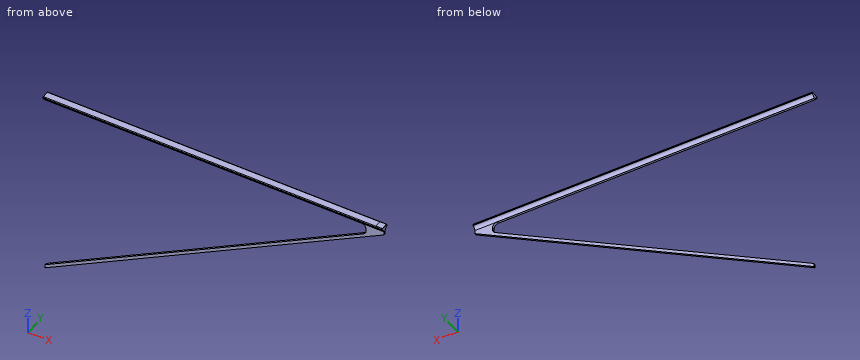
from build123d import *

# Parameters (mm, degrees)
F1_DEPTH      = 502
F3_DEPTH      = 406
F4_DEPTH      = 143
F5_W          = 26.22529459
F5_H          = 3
F6_DEPTH      = 14.25
F6_DEPTH_BACK = 0.8
F8_DEPTH      = 25
F10_DEPTH     = 0.27
F11_R         = 7
F12_R         = 7
F13_T1_DEPTH  = 502
F14_T1_DEPTH  = 502
F15_T1_DEPTH  = 507
F15_T6_DEPTH  = 507
F15_T12_DEPTH = 507
F15_T18_DEPTH = 507
F15_T25_DEPTH = 507
F15_T31_DEPTH = 507


# Not quite as in the source:
# - a fillet or chamfer that OpenCascade refuses, or shapes differently, is made with other operations: its cross-section is extruded or revolved along the edge and cut away or added
# - a feature names something its author has since deleted; it is built from what else it names


with BuildPart() as f1:
    # F0 (on Right) → F1 (new body)
    with BuildSketch(Plane.YZ):
        Polygon((6, 24.6420782059), (-6, 24.6420782059), (-6, 22.1420782059), (-1.5, 22.1420782059), (-1.5, -257.8579217941), (1.5, -257.8579217941), (1.5, 22.1420782059), (6, 22.1420782059), align=None)
    extrude(amount=F1_DEPTH)

    # F2 (on face) → F3 (cut)
    with BuildSketch(Plane.XZ.offset(1.5)):
        Polygon((0, -252.8579217941), (502, 17.1420782059), (0, 17.1420782059), align=None)
    extrude(amount=-F3_DEPTH, mode=Mode.SUBTRACT)

    # F2 (on face) → F4 (cut)
    with BuildSketch(Plane.XZ.offset(1.5)):
        Polygon((502, -257.8579217941), (502, 12.1420782059), (0, -257.8579217941), align=None)
    extrude(amount=-F4_DEPTH, mode=Mode.SUBTRACT)

    # F5 (on face) → F6 (join, two sides)
    with BuildSketch(Plane(origin=(0, 0, 17.1420782059), x_dir=(1, 0, 0), z_dir=(0, 0, -1))) as f6_sk:
        with Locations((488.887352705, 0)):
            Rectangle(F5_W, F5_H)
    extrude(amount=F6_DEPTH)
    extrude(f6_sk.sketch, amount=-F6_DEPTH_BACK)

    # F7 (on face) → F8 (cut)
    with BuildSketch(Plane(origin=(0, 1.5, 0), x_dir=(-1, 0, 0), z_dir=(0, 1, 0))):
        Polygon((-484.8018518519, 2.8920782059), (-502, 12.143202126), (-502, 2.8920782059), align=None)
    extrude(amount=-F8_DEPTH, mode=Mode.SUBTRACT)

    # F9 (on face) → F10 (join)
    with BuildSketch(Plane.XY.offset(24.6420782059)):
        Polygon((501.9800190187, -5.0222751118), (501.9800190187, 4.9777248882), (497.843503952, 4.9777248882), (491.9800190187, 4.9777248882), (491.9800190187, -5.0222751118), (496.5066611767, -5.0222751118), align=None)
    extrude(amount=F10_DEPTH)

    # F11
    f11_edges = [f1.edges().sort_by_distance(p)[0] for p in [
        (475.774705, 0, 17.142078),
    ]]
    fillet(f11_edges, radius=F11_R)

    # F12
    f12_edges = [f1.edges().sort_by_distance(p)[0] for p in [
        (475.774705, 0, 3.03684),
    ]]
    fillet(f12_edges, radius=F12_R)

    # F13: fillet of radius 5 on 1 edges, made by hand

    # F13_s2 → F13_t1 (join)
    with BuildSketch(Plane.YZ):
        with BuildLine():
            ThreePointArc((1.5, 17.1671410204), (2.7919007565, 20.5212429867), (6, 22.1420782059))
            Line((6, 22.1420782059), (1.5, 22.1420782059))
            Line((1.5, 22.1420782059), (1.5, 17.1671410204))
        make_face()
    extrude(amount=F13_T1_DEPTH)

    # F14: fillet of radius 5 on 1 edges, made by hand

    # F14_s2 → F14_t1 (join)
    with BuildSketch(Plane.YZ):
        with BuildLine():
            ThreePointArc((-1.5, 17.1671410204), (-2.7919007565, 20.5212429867), (-6, 22.1420782059))
            Line((-6, 22.1420782059), (-1.5, 22.1420782059))
            Line((-1.5, 22.1420782059), (-1.5, 17.1671410204))
        make_face()
    extrude(amount=F14_T1_DEPTH)

    # F15: fillet of radius 1 on 2 edges, made by hand

    # F15_s2 → F15_t1 (cut)
    with BuildSketch(Plane.YZ.offset(-2.5)):
        with BuildLine():
            ThreePointArc((6, 23.6420782059), (5.7071067812, 24.3491849871), (5, 24.6420782059))
            Line((5, 24.6420782059), (6, 24.6420782059))
            Line((6, 24.6420782059), (6, 23.6420782059))
        make_face()
    extrude(amount=F15_T1_DEPTH, mode=Mode.SUBTRACT)


with BuildPart() as f15_tool4:
    # F15_s5 → F15_t6 (new body)
    with BuildSketch(Plane.YZ.offset(-2.5)):
        with BuildLine():
            ThreePointArc((-5, 24.6420782059), (-5.7071067812, 24.3491849871), (-6, 23.6420782059))
            Line((-6, 23.6420782059), (-6, 24.6420782059))
            Line((-6, 24.6420782059), (-5, 24.6420782059))
        make_face()
    extrude(amount=F15_T6_DEPTH)

    split(bisect_by=Plane.YZ.offset(491.9800190187), keep=Keep.BOTTOM)

    split(bisect_by=Plane.XZ.offset(5.0222751118), keep=Keep.BOTTOM)


with BuildPart() as f1_1:
    add(f1.part)

    # F15_t3: cut F15_tool4
    add(f15_tool4.part, mode=Mode.SUBTRACT)


with BuildPart() as f15_tool10:
    # F15_s11 → F15_t12 (new body)
    with BuildSketch(Plane.YZ.offset(-2.5)):
        with BuildLine():
            ThreePointArc((-5, 24.6420782059), (-5.7071067812, 24.3491849871), (-6, 23.6420782059))
            Line((-6, 23.6420782059), (-6, 24.6420782059))
            Line((-6, 24.6420782059), (-5, 24.6420782059))
        make_face()
    extrude(amount=F15_T12_DEPTH)

    split(bisect_by=Plane.YZ.offset(491.9800190187), keep=Keep.BOTTOM)

    split(bisect_by=Plane.XZ.offset(5.0222751118), keep=Keep.TOP)


with BuildPart() as f1_2:
    add(f1_1.part)

    # F15_t9: cut F15_tool10
    add(f15_tool10.part, mode=Mode.SUBTRACT)


with BuildPart() as f15_tool16:
    # F15_s17 → F15_t18 (new body)
    with BuildSketch(Plane.YZ.offset(-2.5)):
        with BuildLine():
            ThreePointArc((-5, 24.6420782059), (-5.7071067812, 24.3491849871), (-6, 23.6420782059))
            Line((-6, 23.6420782059), (-6, 24.6420782059))
            Line((-6, 24.6420782059), (-5, 24.6420782059))
        make_face()
    extrude(amount=F15_T18_DEPTH)

    split(bisect_by=Plane.YZ.offset(491.9800190187), keep=Keep.TOP)

    split(bisect_by=Plane.YZ.offset(501.9800190187), keep=Keep.BOTTOM)

    split(bisect_by=Plane.XZ.offset(5.0222751118), keep=Keep.TOP)


with BuildPart() as f1_3:
    add(f1_2.part)

    # F15_t15: cut F15_tool16
    add(f15_tool16.part, mode=Mode.SUBTRACT)


with BuildPart() as f15_tool23:
    # F15_s24 → F15_t25 (new body)
    with BuildSketch(Plane.YZ.offset(-2.5)):
        with BuildLine():
            ThreePointArc((-5, 24.6420782059), (-5.7071067812, 24.3491849871), (-6, 23.6420782059))
            Line((-6, 23.6420782059), (-6, 24.6420782059))
            Line((-6, 24.6420782059), (-5, 24.6420782059))
        make_face()
    extrude(amount=F15_T25_DEPTH)

    split(bisect_by=Plane.YZ.offset(501.9800190187), keep=Keep.TOP)

    split(bisect_by=Plane.XZ.offset(5.0222751118), keep=Keep.BOTTOM)


with BuildPart() as f1_4:
    add(f1_3.part)

    # F15_t22: cut F15_tool23
    add(f15_tool23.part, mode=Mode.SUBTRACT)


with BuildPart() as f15_tool29:
    # F15_s30 → F15_t31 (new body)
    with BuildSketch(Plane.YZ.offset(-2.5)):
        with BuildLine():
            ThreePointArc((-5, 24.6420782059), (-5.7071067812, 24.3491849871), (-6, 23.6420782059))
            Line((-6, 23.6420782059), (-6, 24.6420782059))
            Line((-6, 24.6420782059), (-5, 24.6420782059))
        make_face()
    extrude(amount=F15_T31_DEPTH)

    split(bisect_by=Plane.YZ.offset(501.9800190187), keep=Keep.TOP)

    split(bisect_by=Plane.XZ.offset(5.0222751118), keep=Keep.TOP)


with BuildPart() as f1_5:
    add(f1_4.part)

    # F15_t28: cut F15_tool29
    add(f15_tool29.part, mode=Mode.SUBTRACT)


solid = f1_5.part
Could you check a few things on this model? Use its own coordinates, in mm. Round coordinates to 2 decimals unless told otherwise and drop trailing zeros. Order: outer loops, then holes, each group sorted by start corner. A loop starts at its lowest first (then second) coordinate and runs counter-clockwise, first axis right, second up.
(1) Imagine slicing it at B-B (z = -207). Write out the boundary of the cut face in (x, y), plus the area to 3 significant figures.
Response values:
outline: (85.26, -1.5) - (94.56, -1.5) - (94.56, 1.5) - (85.26, 1.5) - close
area: 27.9 mm2
(2) I'm going to push flat-ended pins straight in: pin 1 (1 mm diameter, centred on x = 263, y = -3, fed in from -Z); pin 2 (6 mm diameter, centred on x = 252.5, y = -4, fed in from -Z); pin 3 (1.5 mm diameter, centred on x = 165.5, y = 0.5, fed in from +Z). Where does each tip first touch, or does it pass through?
Response values:
pin 1: stops at z = 20.17
pin 2: stops at z = -122.94
pin 3: stops at z = 24.64
(3) Please list where these lines run through material, in increasing order: line 1 along Y through (x, z) = (413, -35.5); line 2 along Z through (x, y) = (347, -0.75); line 3 along Z through (x, y) = (453, 1.25).
Response values:
line 1: y = -1.5 to 1.5
line 2: z = -71.22 to -66.22, 17.14 to 24.64
line 3: z = -14.21 to -9.21, 17.14 to 24.64
